Geometry check sheet. Reference: the model listing, model coordinates, mm. Face numbers are marked on the shaded views. A direction names the side the tool comes from. Give positions to 0.01 mm unless a question says otherwise; leave off trailing zeros. Loops run counter-clockwise (first coordinate to the right, second up) from the corner with the lowest first, then second, coordinate; pieces in that order, holes last.
1. Tool access check on the marked faces 4, 5 and 6. Record the directions out of +Z, -Z, +X, -X, +Y, -Y that give a thin tool (end or side, any length) a straight path to the whole face; none if there is none.
2. Material ranges on L1, parallel to Y at x = -0.75, z = 1.25; L2, parallel to X at y = 18, z = 0; L3, parallel to Z at x = 1, y = 18.25, recorded low to high.
3. Go/stop test with a flat-tipped pin: pin 1 Ø1 at (x, y) = (0, 11.5) entering from -Z. Record where the tip stops, or that it passes through.
4. Cross-section at C-C, the plane y = 1.5. Record the cut outline in (x, z), plus the area to 3 significant figures.
5. Cross-section at D-D, the plane x = -1.75. Record the cut outline in (y, z).
6. Release check for a two-part mould opening along Z. For the marked faces 1, 2 and 3 record: +Z half, -Z half, draft (parallel to the pull), parting line (faces both ways), or undercut.
7. Cross-section at A-A, the plane x = 2.5. Record the cut outline in (y, z), plus the area to 3 significant figures.
8. Cross-section at B-B, the plane z = 0. Record the cut outline in (x, y).
from build123d import *

# Parameters (mm, degrees)
ESQUISSE1_R             = 2
BOSS_EXTRU_2_DEPTH      = 15
ESQUISSE4_R             = 3.5
BOSS_EXTRU_5_DEPTH      = 5
ENL_V_MAT_EXTRU_3_DEPTH = 4


with BuildPart() as part:
    # Esquisse1 → Boss.-Extru.2 (new body)
    with BuildSketch(Plane(origin=(0, 0, 0), x_dir=(1, 0, 0), z_dir=(0, 1, 0))):
        with Locations(Location((0, 0, 0), (0, 0, 270))):
            Circle(ESQUISSE1_R)
    extrude(amount=BOSS_EXTRU_2_DEPTH)

    # Esquisse4 → Boss.-Extru.5 (add)
    with BuildSketch(Plane(origin=(0, 15, 0), x_dir=(1, 0, 0), z_dir=(0, 1, 0))):
        with Locations(Location((0, 0, 0), (0, 0, 270))):
            Circle(ESQUISSE4_R)
    extrude(amount=BOSS_EXTRU_5_DEPTH)

    # Esquisse6 → Enlèv. mat.-Extru.3 (cut)
    with BuildSketch(Plane(origin=(0, 20, 0), x_dir=(1, 0, 0), z_dir=(0, 1, 0))):
        Polygon((0.539972864, -2.835800176), (2.725861425, -0.950269871), (2.185888561, 1.885530305), (-0.539972864, 2.835800176), (-2.725861425, 0.950269871), (-2.185888561, -1.885530305), align=None)
    extrude(amount=-ENL_V_MAT_EXTRU_3_DEPTH, mode=Mode.SUBTRACT)


solid = part.part
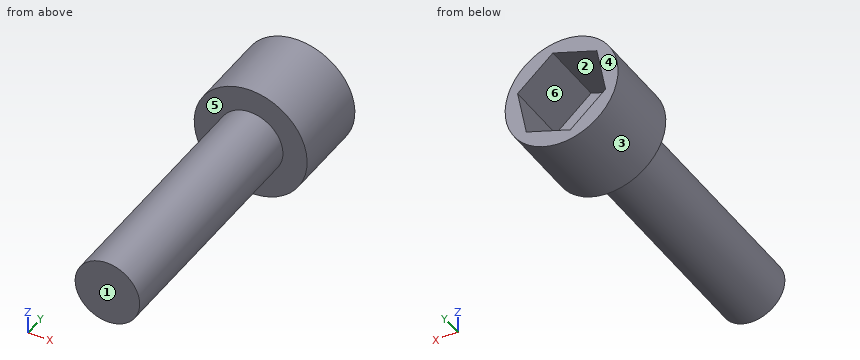
Result:
1. face 4: +Z, -Z, +X, -X, +Y
1. face 5: -Y
1. face 6: +Y
2. L1: y = 0 to 16
2. L2: x = -3.5 to -2.54, 2.54 to 3.5
2. L3: z = -3.35 to -2.3, 2.44 to 3.35
3. pin 1: stops at z = -2
4. outline: circle Ø4 at (0, 0)
4. area: 12.6 mm2
5. outline: (0, -0.97) - (15, -0.97) - (15, -3.03) - (20, -3.03) - (20, -1.79) - (16, -1.79) - (16, 2.04) - (20, 2.04) - (20, 3.03) - (15, 3.03) - (15, 0.97) - (0, 0.97) - close
6. face 1: draft
6. face 2: undercut
6. face 3: parting line
7. outline: (15, -2.45) - (20, -2.45) - (20, -0.24) - (16, -0.24) - (16, 1.15) - (20, 1.15) - (20, 2.45) - (15, 2.45) - close
7. area: 19.0 mm2
8. outline: (-3.5, 15) - (-2, 15) - (-2, 0) - (2, 0) - (2, 15) - (3.5, 15) - (3.5, 20) - (2.54, 20) - (2.54, 16) - (-2.54, 16) - (-2.54, 20) - (-3.5, 20) - close
